Can you work these out from the model? Positions are in its coordinate system, mm. Face numbers are marked on the shaded views. A direction names the side the tool comes from. Coordinates: 2 decimals unless noted, no trailing zeros. Order: outer loops, then holes, each group sorted by start corner. A loop starts at its lowest first (then second) coordinate and runs counter-clockwise, first axis right, second up. Notation, with made-up numbers: M -6.5,-28.75 L 18.5,-28.75 A30 ccw 18.5,-4.75 Z; hole C -4,-32.75 d9. An arc over 180 degrees is marked long. Answer as CSV lines item,"result". Start each with the question number.
1. Will these pins go through, and if not, where does the flat tip stop? pin 1 (10.5 mm diameter, centred on y = -15, z = 13.5, fed in from -X); pin 2 (6.5 mm diameter, centred on x = -25.5, z = 19, fed in from +Y); pin 3 (17 mm diameter, centred on y = -17, z = 20.5, fed in from +X); pin 4 (23.5 mm diameter, centred on y = -11.5, z = -17, fed in from -X).
2. If we section it at B-B (y = 7.5): List the corners of the cut face in (x, z) for me, plus the area to 3 significant figures.
3. If we section it at D-D (y = -11): List the corners of the cut face in (x, z) for me.
4. If we mould it in two halves opening along X, with no side actions, what happens to the marked faces 1, 2 and 3? For each: released by +X, released by -X, zero draft, split by the parting line, or undercut.
5. If we section it at A-A (z = -3): List the corners of the cut face in (x, y) for me.
6. If we section it at C-C (x = -29): List the corners of the cut face in (y, z) for me.
7. On a 3-axis mill with a long thin cutter (end or side, diameter ignored), from which of +Z, -Z, +X, -X, +Y, -Y can I reach the whole of each face in a straight line? I mean the marked faces 4, 5 and 6. Say none if no direction works.
8. I need wall thicknesses on line 1 along Y through (x, z) = (-32, 9); line 2 along X through (y, z) = (12, 3); line 3 along X through (y, z) = (14, -10.5). Which ranges of each line are inside material? Lowest first, please. Write a range as from..to.
```python
from build123d import *

# Parameters (mm, degrees)
BOSS_EXTRUDE2_DEPTH = 26
RIB1_REACH          = 60.322
SKETCH5_WALL_W      = 164.701059438
SKETCH5_WALL_H      = 8


with BuildPart() as part:
    # Sketch3 → Boss-Extrude2 (new, symmetric)
    with BuildSketch(Plane.XY):
        with BuildLine():
            Line((-37.5, -27.321428571), (-4.5, -27.321428571))
            Line((-4.5, -27.321428571), (-4.5, -6.162629994))
            ThreePointArc((-4.5, -6.162629994), (-17.783419244, 1.806904997), (-23, 16.392857143))
            Line((-23, 16.392857143), (-15, 16.392857143))
            ThreePointArc((-15, 16.392857143), (0, 1.392857143), (15, 16.392857143))
            Line((15, 16.392857143), (23, 16.392857143))
            ThreePointArc((23, 16.392857143), (17.783419244, 1.806904997), (4.5, -6.162629994))
            Line((4.5, -6.162629994), (4.5, -27.321428571))
            Line((4.5, -27.321428571), (37.5, -27.321428571))
            Line((37.5, -27.321428571), (37.5, -36.321428571))
            Line((37.5, -36.321428571), (-37.5, -36.321428571))
            Line((-37.5, -36.321428571), (-37.5, -27.321428571))
        make_face()
    extrude(amount=BOSS_EXTRUDE2_DEPTH, both=True)

    # Sketch5 wall → Rib1 (add, up to next)
    with BuildSketch(Plane(origin=(30.25, -5.464285714, 0), x_dir=(0.314831618537, -0.949147539622, 0), z_dir=(0.949147539622, 0.314831618537, 0)), mode=Mode.PRIVATE) as rib1_sk1:
        Rectangle(SKETCH5_WALL_W, SKETCH5_WALL_H)
    rib1_tool1 = extrude(rib1_sk1.sketch, amount=-RIB1_REACH, mode=Mode.PRIVATE) - part.part
    rib1 = rib1_tool1.solids().sort_by_distance((30.25, -5.464285714, 0))[0]
    add(rib1)

    # Mirror1: Rib1 across plane
    add(rib1.mirror(Plane(origin=(0, 0, 0), x_dir=(0, 0, 1), z_dir=(1, 0, 0))))


solid = part.part
```
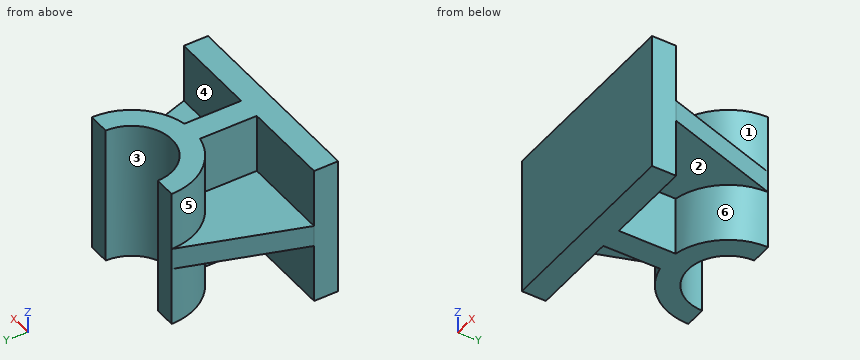
Solved:
1,pin 1,"x = -4.5"
1,pin 2,"y = 16.39"
1,pin 3,"x = 4.5"
1,pin 4,"x = -16.38"
2,outline,"M -25.95,-4 L -21.21,-4 L -21.21,-26 L -12.08,-26 L -12.08,26 L -21.21,26 L -21.21,4 L -25.95,4 Z; M 12.08,-26 L 21.21,-26 L 21.21,-4 L 25.95,-4 L 25.95,4 L 21.21,4 L 21.21,26 L 12.08,26 Z"
2,area,"1,030 mm²"
3,outline,"M -32.09,-4 L -4.5,-4 L -4.5,-26 L 4.5,-26 L 4.5,-4 L 32.09,-4 L 32.09,4 L 4.5,4 L 4.5,26 L -4.5,26 L -4.5,4 L -32.09,4 Z"
4,face 1,"released by +X"
4,face 2,"zero draft"
4,face 3,"undercut"
5,outline,"M -37.5,-36.32 L 37.5,-36.32 L 37.5,-27.32 L 23,16.39 L 15,16.39 A15 cw -15,16.39 L -23,16.39 L -37.5,-27.32 Z"
6,outline,"M -36.32,-26 L -27.32,-26 L -27.32,-4 L -1.7,-4 L -1.7,4 L -27.32,4 L -27.32,26 L -36.32,26 Z"
7,face 4,"+Z, +X"
7,face 5,"+Z, -X"
7,face 6,"-Z, +X"
8,line 1,"-36.32..-27.32"
8,line 2,"-24.46..-14.34, 14.34..24.46"
8,line 3,"-22.88..-14.81, 14.81..22.88"
